from build123d import *
from build123d.topology import SkipClean

# Parameters (mm, degrees)
SKETCH1_R           = 60
BOSS_EXTRUDE1_DEPTH = 10
SKETCH1_3_R         = 6
BOSS_EXTRUDE2_DEPTH = 10
CUT_EXTRUDE1_START  = -10
CUT_EXTRUDE1_DEPTH  = 10
BOSS_EXTRUDE4_START = 3
SKETCH3_R           = 15
SKETCH3_R_2         = 10
BOSS_EXTRUDE4_DEPTH = 3
FILLET1_R           = 3
CHAMFER1_SIZE       = 0.5


with BuildPart() as part:
    # Sketch1 → Boss-Extrude1 (new body)
    with BuildSketch(Plane.XY):
        Circle(SKETCH1_R)
    extrude(amount=-BOSS_EXTRUDE1_DEPTH)

    # Sketch1<3> → Boss-Extrude2 (add)
    with BuildSketch(Plane.XY):
        with Locations((-50, 0)):
            Circle(SKETCH1_3_R)
    extrude(amount=BOSS_EXTRUDE2_DEPTH)

    # Sketch2 → Cut-Extrude1 (cut)
    with SkipClean():  # the faces are left unmerged after this step: merging them gives an invalid solid
        with BuildSketch(Plane.XY.offset(CUT_EXTRUDE1_START)):
            with BuildLine():
                ThreePointArc((-14.672214011, -3.118675362), (-14.917828431, -1.567926949), (-15, 0))
                Line((-15, 0), (-44, 0))
                ThreePointArc((-44, 0), (-45.631934066, -4.11339276), (-49.64, -5.989190262))
                ThreePointArc((-49.64, -5.989190262), (-49.322921706, -8.200572806), (-48.907380037, -10.395584541))
                Line((-48.907380037, -10.395584541), (-14.672214011, -3.118675362))
            make_face()
            with BuildLine():
                Line((-44, 0), (-15, 0))
                ThreePointArc((-15, 0), (-14.917828431, 1.567926949), (-14.672214011, 3.118675362))
                Line((-14.672214011, 3.118675362), (-48.907380037, 10.395584541))
                ThreePointArc((-48.907380037, 10.395584541), (-49.322921706, 8.200572806), (-49.64, 5.989190262))
                ThreePointArc((-49.64, 5.989190262), (-45.631934066, 4.11339276), (-44, 0))
            make_face()
            with BuildLine():
                Line((-25, 43.301270189), (-7.5, 12.990381057))
                ThreePointArc((-7.5, 12.990381057), (-4.635254916, 14.265847744), (-1.567926949, 14.917828431))
                Line((-1.567926949, 14.917828431), (-5.226423163, 49.726094768))
                ThreePointArc((-5.226423163, 49.726094768), (-15.450849719, 47.552825815), (-25, 43.301270189))
            make_face()
            with BuildLine():
                ThreePointArc((10.036959095, 11.147172382), (12.135254916, 8.816778784), (13.703181865, 6.101049646))
                Line((13.703181865, 6.101049646), (45.677272882, 20.336832154))
                ThreePointArc((45.677272882, 20.336832154), (40.450849719, 29.389262615), (33.456530318, 37.157241274))
                Line((33.456530318, 37.157241274), (10.036959095, 11.147172382))
            make_face()
            with BuildLine():
                ThreePointArc((13.703181865, -6.101049646), (12.135254916, -8.816778784), (10.036959095, -11.147172382))
                Line((10.036959095, -11.147172382), (33.456530318, -37.157241274))
                ThreePointArc((33.456530318, -37.157241274), (40.450849719, -29.389262615), (45.677272882, -20.336832154))
                Line((45.677272882, -20.336832154), (13.703181865, -6.101049646))
            make_face()
            with BuildLine():
                ThreePointArc((-1.567926949, -14.917828431), (-4.635254916, -14.265847744), (-7.5, -12.990381057))
                Line((-7.5, -12.990381057), (-25, -43.301270189))
                ThreePointArc((-25, -43.301270189), (-15.450849719, -47.552825815), (-5.226423163, -49.726094768))
                Line((-5.226423163, -49.726094768), (-1.567926949, -14.917828431))
            make_face()
        extrude(amount=CUT_EXTRUDE1_DEPTH, mode=Mode.SUBTRACT)

    # Sketch3 → Boss-Extrude4 (add)
    with SkipClean():  # the faces are left unmerged after this step: merging them gives an invalid solid
        with BuildSketch(Plane(origin=(0, 0, -10), x_dir=(-1, 0, 0), z_dir=(0, 0, -1)).offset(BOSS_EXTRUDE4_START)):
            with Locations(Location((0, 0, 0), (0, 0, 156))):
                Circle(SKETCH3_R)
            Circle(SKETCH3_R_2, mode=Mode.SUBTRACT)
        extrude(amount=-BOSS_EXTRUDE4_DEPTH)

    # Fillet1
    # the kernel refuses this fillet: 3 mm, written as the material it takes off along each edge
    with BuildSketch(Plane(origin=(-50, 0, -10), x_dir=(-0.9290450691294319, 0.3699665654167807, 0), z_dir=(-0.3699665654167807, -0.9290450691294319, 0))) as fillet1_piece_1_section:
        with BuildLine():
            CenterArc((6 - FILLET1_R, -FILLET1_R), FILLET1_R, 0, 90)
            Line((6, -FILLET1_R), (6, 0))
            Line((6, 0), (6 - FILLET1_R, 0))
        make_face()
    fillet1_piece_1 = revolve(axis=Axis((-50, 0, -10), (0, 0, -1)), revolution_arc=316.572889398, mode=Mode.PRIVATE)
    fillet1_piece_1 = fillet1_piece_1 & Plane(origin=(0, 0, -9.144891987), x_dir=(-0.9928000000000012, -0.1197838052492802, 0), z_dir=(0, 0, -1)) * Cylinder(50, 24, mode=Mode.PRIVATE)
    add(fillet1_piece_1, mode=Mode.SUBTRACT)

    # Chamfer1
    chamfer1_edges = [part.edges().sort_by_distance(p)[0] for p in [
        (-56, 0, 10),
    ]]
    chamfer(chamfer1_edges, length=CHAMFER1_SIZE)


solid = part.part
Could you check a few things on this model? Use its own coordinates, in mm. A direction names the side the tool comes from. Round coordinates to 2 decimals unless told otherwise and drop trailing zeros. Loops run counter-clockwise (first coordinate to the right, second up) from the corner with the lowest first, then second, coordinate; pieces in that order, holes last. Notation, with made-up numbers: (34.5, -24) - (66.5, -24) arc R36 cw to (66.5, 15) - close; hole circle Ø8 at (84, -6). An arc over 180 degrees is marked (long way). Write item = value, one per line.
1) Imagine slicing it at B-B (x = 0). Please give me the cut outline in (y, z), and give its area (3 significant figures).
Computed:
outline = (-60, -10) - (-15, -10) - (-15, -13) - (-10, -13) - (-10, -10) - (10, -10) - (10, -13) - (15, -13) - (15, -10) - (60, -10) - (60, 0) - (-60, 0) - close
area = 1,230 mm2
2) If we mould it in two halves opening along X, with no side actions, what happens to faces 1 (the cylindrical face through (40, -30, -5)), 2 (the flat face through (-1.1, 10.2, -13)), 3 (the cylindrical face through (-59.94, 2.64, -4.93))? For each: pulls with the +X half, pulls with the -X half, needs draft (parallel to the pull), parting line crosses it, or undercut.
Computed:
face_1 = undercut
face_2 = needs draft
face_3 = parting line crosses it
3) On a 3-axis mill with a long thin cutter (end or side, diameter ignored), from which of +Z, -Z, +X, -X, +Y, -Y can I reach the whole of each face in a straight line? I mean faces 4 (the cylindrical face through (40.537, 29.271, -5.07)), 5 (the flat face through (-50, 0, 10)), 6 (the flat face through (-14, -12, -10)). Say none if no direction works.
Computed:
face_4 = +Z, -Z
face_5 = +Z, +X, -X, +Y, -Y
face_6 = -Z
4) I need wall thicknesses on line 1 along Y through (x, z) = (0, -11.65); line 2 along X through (y, z) = (-15, -4); line 3 along Z through (x, y) = (16, 29). Which ranges of each line are inside material? Lowest first, please. Write a range as from..to.
Computed:
line_1 = -15..-10, 10..15
line_2 = -58.09..-8.66, -1.58..13.51, 33.69..58.09
line_3 = -10..0
5) I'm going to push flat-ended pins straight in: P1, Ø1.5, axis at x = -27.5, y = -10.5, coming from the +Z side; P2, Ø3, axis at y = -3, z = -9, coming from the -X side; P3, Ø10, axis at x = 4.5, z = 0, coming from the -Y side. Where does each tip first touch, or does it pass through?
Computed:
P1 = 0
P2 = -59.98
P3 = -60
6) Imagine slicing it at C-C (y = 28.5). Please give me the cut outline in (x, z).
Computed:
outline = (-52.8, -10) - (-16.45, -10) - (-16.45, 0) - (-52.8, 0) - close; (-3, -10) - (25.66, -10) - (25.66, 0) - (-3, 0) - close; (41.08, -10) - (52.8, -10) - (52.8, 0) - (41.08, 0) - close
7) Imagine slicing it at A-A (x = -41.5). Please give me the cut outline in (y, z).
Computed:
outline = (-43.33, -10) - (-8.82, -10) - (-8.82, 0) - (-43.33, 0) - close; (8.82, -10) - (43.33, -10) - (43.33, 0) - (8.82, 0) - close
8) Imagine slicing it at D-D (z = 2). Please give me the cut outline in (x, y), and give its area (3 significant figures).
Computed:
outline = circle Ø12 at (-50, 0)
area = 113 mm2
